```python
from build123d import *

# Parameters (mm, degrees)
SKETCH1_W                   = 50.8
SKETCH1_H                   = 101.6
BOSS_EXTRUDE2_DEPTH         = 2.54
F_1_4_0_25_DIAMETER_HOLE1_D = 6.35
SKETCH5_W                   = 2.54
SKETCH5_H                   = 25.4
BOSS_EXTRUDE3_REACH         = 116.046
BOSS_EXTRUDE3_END_RADIUS    = 6.35
SKETCH6_W                   = 2.54
SKETCH6_H                   = 25.4
SKETCH7_W                   = 2.54
SKETCH7_H                   = 21.59
BOSS_EXTRUDE4_REACH         = 116.05
BOSS_EXTRUDE4_END_RADIUS    = 6.395590949
SKETCH8_W                   = 2.54
SKETCH8_H                   = 21.59
BOSS_EXTRUDE5_START         = -2.54
SKETCH9_R                   = 6.35
BOSS_EXTRUDE5_DEPTH         = 2.54


with BuildPart() as part:
    # Sketch1 → Boss-Extrude2 (new body)
    with BuildSketch(Plane.XY):
        with Locations((25.4, 50.8)):
            Rectangle(SKETCH1_W, SKETCH1_H)
    extrude(amount=-BOSS_EXTRUDE2_DEPTH)

    # 1/4 (0.25) Diameter Hole1 (through all)
    with Locations(Plane(origin=(25.4, 76.2, 0), x_dir=(1, 0, 0), z_dir=(0, 0, 1))):
        with Locations((0, 0), (-0.127319097, -50.8), (0, -25.4)):
            Hole(F_1_4_0_25_DIAMETER_HOLE1_D / 2)



with BuildPart() as body_2:
    # Sketch5 → Revolve2 (revolve)
    with BuildSketch(Plane.XY.offset(-1.27), mode=Mode.PRIVATE) as revolve2_sk:
        with Locations((-1.27, 88.9)):
            Rectangle(SKETCH5_W, SKETCH5_H)
    revolve(revolve2_sk.sketch.rotate(Axis((-8.89, 0, -1.27), (0, 1, 0)), 90), axis=Axis((-8.89, 0, -1.27), (0, 1, 0)))


with BuildPart() as part_1:
    add(part.part)

    add(body_2.part)  # Boss-Extrude3 merges body 2
    # Boss-Extrude3: up to this cylinder (the profile starts outside it)
    boss_extrude3_end = Plane(origin=(-8.89, 88.9, -1.27), z_dir=(0, -1, 0)) * Cylinder(BOSS_EXTRUDE3_END_RADIUS, 245.792, mode=Mode.PRIVATE)
    # Sketch6 → Boss-Extrude3 (add, up to the surface)
    with BuildSketch(Plane.ZY, mode=Mode.PRIVATE) as boss_extrude3_sk1:
        with Locations((-1.27, 88.9)):
            Rectangle(SKETCH6_W, SKETCH6_H)
    boss_extrude3_tool1 = extrude(boss_extrude3_sk1.sketch, amount=BOSS_EXTRUDE3_REACH, mode=Mode.PRIVATE) - boss_extrude3_end
    add(boss_extrude3_tool1.solids().sort_by_distance((0, 88.9, -1.27))[0])



with BuildPart() as body_2_2:
    # Sketch7 → Revolve3 (revolve)
    with BuildSketch(Plane.XY.offset(-1.27), mode=Mode.PRIVATE) as revolve3_sk:
        with Locations((-1.27, 38.735)):
            Rectangle(SKETCH7_W, SKETCH7_H)
    revolve(revolve3_sk.sketch.rotate(Axis((-8.935590949, 101.6, -1.27), (0, -1, 0)), 180), axis=Axis((-8.935590949, 101.6, -1.27), (0, -1, 0)))


with BuildPart() as part_2:
    add(part_1.part)

    add(body_2_2.part)  # Boss-Extrude4 merges body 2 2
    # Boss-Extrude4: up to this cylinder (the profile starts outside it)
    boss_extrude4_end = Plane(origin=(-8.935590949, 38.735, -1.27), z_dir=(0, 1, 0)) * Cylinder(BOSS_EXTRUDE4_END_RADIUS, 245.891181898, mode=Mode.PRIVATE)
    # Sketch8 → Boss-Extrude4 (add, up to the surface)
    with BuildSketch(Plane.ZY, mode=Mode.PRIVATE) as boss_extrude4_sk1:
        with Locations((-1.27, 38.735)):
            Rectangle(SKETCH8_W, SKETCH8_H)
    boss_extrude4_tool1 = extrude(boss_extrude4_sk1.sketch, amount=BOSS_EXTRUDE4_REACH, mode=Mode.PRIVATE) - boss_extrude4_end
    add(boss_extrude4_tool1.solids().sort_by_distance((0, 38.735, -1.27))[0])

    # Sketch9 → Boss-Extrude5 (add)
    with BuildSketch(Plane(origin=(0, 101.6, 0), x_dir=(1, 0, 0), z_dir=(0, 1, 0)).offset(BOSS_EXTRUDE5_START)):
        with Locations(Location((-8.89, 1.27, 0), (0, 0, 90))):
            Circle(SKETCH9_R)
    extrude(amount=BOSS_EXTRUDE5_DEPTH)


solid = part_2.part
```
Geometry: final body of the model. Coordinates: model frame, mm. A direction names the side the tool comes from. Coordinates: 2 decimals unless noted, no trailing zeros. Order: outer loops, then holes, each group sorted by start corner. A loop starts at its lowest first (then second) coordinate and runs counter-clockwise, first axis right, second up. Notation, with made-up numbers: (61, 45) -> (65, 45) arc R15 cw to (65, 55) -> close; hole circle Ø4 at (73, 82.25). An arc over 180 degrees is marked (long way). Write each question's results on one line, items separated by ' | '. Start each with the question number.
1) First-contact query: pin 1 (5 mm diameter, centred on x = 37.5, y = 11, fed in from +Z); pin 2 (6 mm diameter, centred on x = 28.5, y = 22.5, fed in from -Z); pin 3 (5.5 mm diameter, centred on x = -9.5, z = -1.5, fed in from -Y). Flat tips, straight axial feed; report the tip coordinate or a pass-through.
2) Cut plane C-C, the plane x = -4. Output: boundary loops of the cut face in (y, z).
3) Set-up query: faces 1 (the flat face through (-9, 99.06, -1)), 2 (the flat face through (0, 14, -1)), 3 (the flat face through (19, 52, 0)), 4 (the flat face through (31, 50, -2.54)), 5 (the flat face through (0, 63, -1)). Return all of +Z, -Z, +X, -X, +Y, -Y with unobstructed straight access to the full face (end or side cutting, diameter ignored); none if empty.
4) Cut plane A-A, the plane y = 50.8. Output: boundary loops of the cut face in (x, z) (3 decimals).
5) Cut plane D-D, the plane x = 9.5. Output: boundary loops of the cut face in (y, z).
6) Cut plane B-B, the plane x = 25.4. Output: boundary loops of the cut face in (y, z) (3 decimals), and give its area (3 significant figures).
7) Material intervals for line 1 along Y through (x, z) = (25.4, -1.65) (3 decimals); line 2 along X through (y, z) = (86.25, -1.27); line 3 along Y through (x, z) = (-2, -1.5), sorted ascending.
8) Mould query, pull axis Z, two halves, no side actions, for faces 6 (the cylindrical face through (23.693, 53.477, -1.288)), 7 (the cylindrical face through (-17.772, 89.078, -1.643)), 8 (the cylindrical face through (-2.6, 87.5, -0.4)). Classes: released by +Z, released by -Z, zero draft, split by the parting line, or undercut.
Checks:
1) pin 1: z = 0 | pin 2: z = -2.54 | pin 3: y = 99.06
2) outline: (27.94, -8.72) -> (49.53, -8.72) -> (49.53, -5.34) -> (27.94, -5.34) -> close; (27.94, 2.8) -> (49.53, 2.8) -> (49.53, 6.18) -> (27.94, 6.18) -> close; (76.2, -8.69) -> (101.6, -8.69) -> (101.6, 6.15) -> (76.2, 6.15) -> (76.2, 2.78) -> (99.06, 2.78) -> (99.06, -5.32) -> (76.2, -5.32) -> close
3) face 1: -Y | face 2: +Z, -Z, -X, -Y | face 3: +Z, +X, +Y, -Y | face 4: -Z, +X, +Y, -Y | face 5: +Z, -Z, -X
4) outline: (0, -2.54) -> (22.225, -2.54) -> (22.225, 0) -> (0, 0) -> close; (28.575, -2.54) -> (50.8, -2.54) -> (50.8, 0) -> (28.575, 0) -> close
5) outline: (0, -2.54) -> (101.6, -2.54) -> (101.6, 0) -> (0, 0) -> close
6) outline: (0, -2.54) -> (22.228, -2.54) -> (22.228, 0) -> (0, 0) -> close; (28.572, -2.54) -> (47.625, -2.54) -> (47.625, 0) -> (28.572, 0) -> close; (53.975, -2.54) -> (73.025, -2.54) -> (73.025, 0) -> (53.975, 0) -> close; (79.375, -2.54) -> (101.6, -2.54) -> (101.6, 0) -> (79.375, 0) -> close | area: 210 mm^2
7) line 1: 0 to 22.228, 28.572 to 47.625, 53.975 to 73.025, 79.375 to 101.6 | line 2: -17.78 to -15.24, -2.54 to 50.8 | line 3: 27.94 to 49.53, 76.2 to 101.6
8) face 6: zero draft | face 7: split by the parting line | face 8: undercut
